Part model, mm, in its own coordinate system. Face numbers are marked on the shaded views. Round coordinates to 2 decimals unless told otherwise and drop trailing zeros. Return JSON: item names as keys, results as strings. Group by question number.
Item 1: Two-plate mould, pull along Y, no slides. Class the marked faces 1 and 2: released by +Y, released by -Y, zero draft, split by the parting line, or undercut.
Item 2: Probe probe 1 along X at (y, z) = (0.85, 17.5). List the from-to ranges inside material, lowest first.
Item 3: Drop flat-ended pins along their axis: pin 1 (6.5 mm diameter, centred on x = -110.93, z = 17.5, fed in from -Y); pin 2 (8 mm diameter, centred on x = -110.93, z = -17.5, fed in from +Y). Give the stop position or say it passes through.
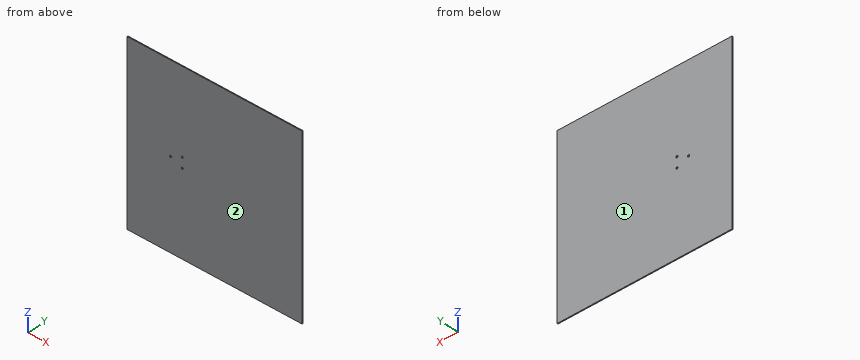
```python
from build123d import *

# Parameters (mm, degrees)
SKETCH1_W               = 600
SKETCH1_H               = 600
BOSS_EXTRUDE1_DEPTH     = 3
CUT_EXTRUDE1_DEPTH      = 425.274675181
CUT_EXTRUDE1_DEPTH_BACK = 425.274675181
SKETCH2_R               = 3.5
CUT_EXTRUDE2_DEPTH      = 425.274675181
CUT_EXTRUDE2_DEPTH_BACK = 425.274675181
SKETCH3_R               = 3.55


with BuildPart() as part:
    # Sketch1 → Boss-Extrude1 (new body)
    with BuildSketch(Plane(origin=(0, 0, 0), x_dir=(1, 0, 0), z_dir=(0, 1, 0))):
        Rectangle(SKETCH1_W, SKETCH1_H)
    extrude(amount=BOSS_EXTRUDE1_DEPTH)

    # Sketch2 → Cut-Extrude1 (cut, two sides: drawn at the far end of the back side and taken through both)
    with BuildSketch(Plane(origin=(0, 3, 0), x_dir=(1, 0, 0), z_dir=(0, 1, 0)).offset(-CUT_EXTRUDE1_DEPTH_BACK)):
        with Locations(Location((-110.928868976, -17.5, 0), (0, 0, 270))):
            Circle(SKETCH2_R)
        with Locations(Location((-110.928868976, 17.5, 0), (0, 0, 270))):
            Circle(SKETCH2_R)
    extrude(amount=CUT_EXTRUDE1_DEPTH + CUT_EXTRUDE1_DEPTH_BACK, mode=Mode.SUBTRACT)

    # Sketch3 → Cut-Extrude2 (cut, two sides: drawn at the far end of the back side and taken through both)
    with BuildSketch(Plane(origin=(0, 3, 0), x_dir=(1, 0, 0), z_dir=(0, 1, 0)).offset(-CUT_EXTRUDE2_DEPTH_BACK)):
        with Locations(Location((-150.928868976, 0, 0), (0, 0, 270))):
            Circle(SKETCH3_R)
    extrude(amount=CUT_EXTRUDE2_DEPTH + CUT_EXTRUDE2_DEPTH_BACK, mode=Mode.SUBTRACT)


solid = part.part
```
Filled in:
{
 "1": {"face 1": "released by +Y", "face 2": "released by -Y"},
 "2": {"probe 1": "x = -300 to -114.43, -107.43 to 300"},
 "3": {"pin 1": "passes through", "pin 2": "stops at y = 3"}
}
